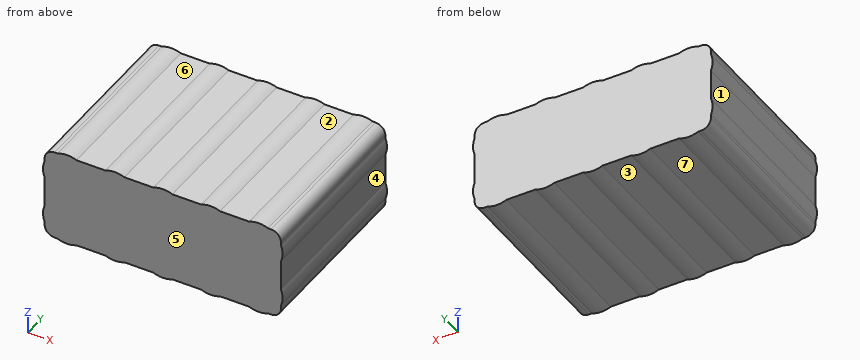
```python
from build123d import *

# Parameters (mm, degrees)
BOSS_EXTRUDE1_DEPTH = 54


with BuildPart() as part:
    # Sketch1 → Boss-Extrude1 (new body)
    with BuildSketch(Plane(origin=(0, 0, 0), x_dir=(1, 0, 0), z_dir=(0, 1, 0))):
        with BuildLine():
            ThreePointArc((-34.630594518, -14.480554015), (-33.751914861, -16.601874359), (-31.630594518, -17.480554015))
            Line((-31.630594518, -17.480554015), (-30.728869867, -17.480554015))
            ThreePointArc((-30.728869867, -17.480554015), (-27.830594518, -18.080554015), (-24.932319169, -17.480554015))
            Line((-24.932319169, -17.480554015), (-16.128869867, -17.480554015))
            ThreePointArc((-16.128869867, -17.480554015), (-13.230594518, -18.080554015), (-10.332319169, -17.480554015))
            Line((-10.332319169, -17.480554015), (-1.528869867, -17.480554015))
            ThreePointArc((-1.528869867, -17.480554015), (1.369405482, -18.080554015), (4.267680831, -17.480554015))
            Line((4.267680831, -17.480554015), (13.071130133, -17.480554015))
            ThreePointArc((13.071130133, -17.480554015), (15.969405482, -18.080554015), (18.867680831, -17.480554015))
            Line((18.867680831, -17.480554015), (27.671130133, -17.480554015))
            ThreePointArc((27.671130133, -17.480554015), (30.569405482, -18.080554015), (33.467680831, -17.480554015))
            Line((33.467680831, -17.480554015), (34.369405482, -17.480554015))
            ThreePointArc((34.369405482, -17.480554015), (36.490725826, -16.601874359), (37.369405482, -14.480554015))
            Line((37.369405482, -14.480554015), (37.369405482, -13.435737625))
            ThreePointArc((37.369405482, -13.435737625), (37.869405482, -10.780554015), (37.369405482, -8.125370406))
            Line((37.369405482, -8.125370406), (37.369405482, 1.164262375))
            ThreePointArc((37.369405482, 1.164262375), (37.869405482, 3.819445985), (37.369405482, 6.474629594))
            Line((37.369405482, 6.474629594), (37.369405482, 7.519445985))
            ThreePointArc((37.369405482, 7.519445985), (36.490725826, 9.640766328), (34.369405482, 10.519445985))
            Line((34.369405482, 10.519445985), (33.467680831, 10.519445985))
            ThreePointArc((33.467680831, 10.519445985), (30.569405482, 11.119445985), (27.671130133, 10.519445985))
            Line((27.671130133, 10.519445985), (18.867680831, 10.519445985))
            ThreePointArc((18.867680831, 10.519445985), (15.969405482, 11.119445985), (13.071130133, 10.519445985))
            Line((13.071130133, 10.519445985), (4.267680831, 10.519445985))
            ThreePointArc((4.267680831, 10.519445985), (1.369405482, 11.119445985), (-1.528869867, 10.519445985))
            Line((-1.528869867, 10.519445985), (-10.332319169, 10.519445985))
            ThreePointArc((-10.332319169, 10.519445985), (-13.230594518, 11.119445985), (-16.128869867, 10.519445985))
            Line((-16.128869867, 10.519445985), (-24.932319169, 10.519445985))
            ThreePointArc((-24.932319169, 10.519445985), (-27.830594518, 11.119445985), (-30.728869867, 10.519445985))
            Line((-30.728869867, 10.519445985), (-31.630594518, 10.519445985))
            ThreePointArc((-31.630594518, 10.519445985), (-33.751914861, 9.640766328), (-34.630594518, 7.519445985))
            Line((-34.630594518, 7.519445985), (-34.630594518, 6.474629594))
            ThreePointArc((-34.630594518, 6.474629594), (-35.130594518, 3.819445985), (-34.630594518, 1.164262375))
            Line((-34.630594518, 1.164262375), (-34.630594518, -8.125370406))
            ThreePointArc((-34.630594518, -8.125370406), (-35.130594518, -10.780554015), (-34.630594518, -13.435737625))
            Line((-34.630594518, -13.435737625), (-34.630594518, -14.480554015))
        make_face()
    extrude(amount=BOSS_EXTRUDE1_DEPTH)


solid = part.part
```
Check sheet for the modelled part. Datum: model origin and axes. Units: mm. Face numbers are marked on the shaded views. A direction names the side the tool comes from. Round coordinates to 2 decimals unless told otherwise and drop trailing zeros. Order: outer loops, then holes, each group sorted by start corner. A loop starts at its lowest first (then second) coordinate and runs counter-clockwise, first axis right, second up. Notation, with made-up numbers: (83.5, 49.5) - (109.5, 49.5) arc R23 cw to (109.5, 74.5) - close; hole circle Ø9 at (19.25, -28.5). An arc over 180 degrees is marked (long way). Answer as CSV lines item,"result". Start each with the question number.
1) Section check A-A (x = -22). Record the cut outline in (y, z).
2) Scan lines: probe 1 along X at (y, z) = (21.5, -0.5); probe 2 along Z at (x, y) = (27, 36); probe 3 along Z at (x, y) = (14, 32). Record each from-to range of solid material in increasing order.
3) Tool access check on the marked faces 5, 6 and 7. Record the directions out of +Z, -Z, +X, -X, +Y, -Y that give a thin tool (end or side, any length) a straight path to the whole face; none if there is none.
4) Draft check along Z on the marked faces 1, 2, 3 and 4. Enter one of: +Z half, -Z half, draft (parallel to the pull), parting line (faces both ways), or undercut.
5) Depth check by flat-ended pin: pin 1 (1.5 mm diameter, centred on y = 13, z = -6, fed in from -X); pin 2 (0.7 mm diameter, centred on x = 34, y = 17.5, fed in from +Z); pin 3 (1 mm diameter, centred on x = -31, y = 33.5, fed in from -Z). Enter the tip coordinate at first touch or a pass-through.
Determined:
1,outline,"(0, -10.52) - (54, -10.52) - (54, 17.48) - (0, 17.48) - close"
2,probe 1,"-34.63 to 37.37"
2,probe 2,"-10.52 to 17.48"
2,probe 3,"-10.85 to 17.81"
3,face 5,"+Z, -Z, +X, -X, -Y"
3,face 6,"+Z, +Y, -Y"
3,face 7,"-Z, +Y, -Y"
4,face 1,"undercut"
4,face 2,"+Z half"
4,face 3,"-Z half"
4,face 4,"undercut"
5,pin 1,"x = -34.99"
5,pin 2,"z = 17.48"
5,pin 3,"z = -10.61"
